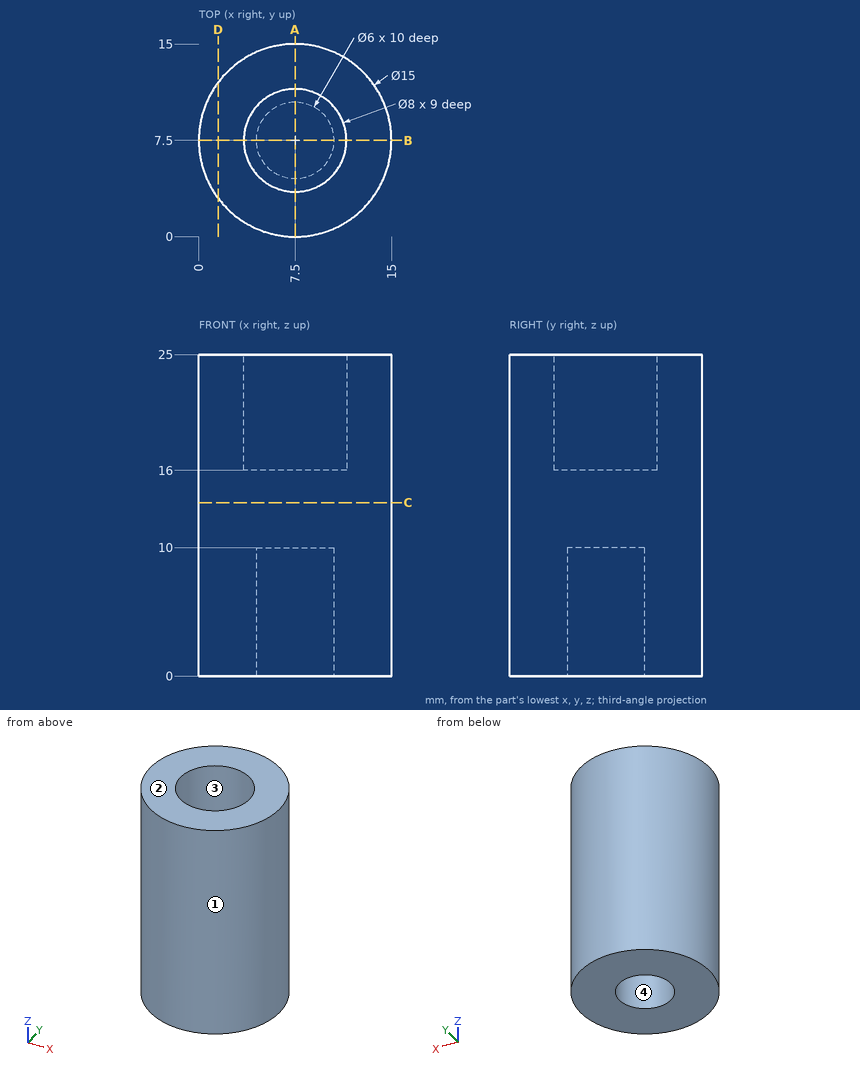
Design review of the part shown in the three views and the two pictorial views. Dimensions are in mm from the part's minimum x, y and z. Give positions to 0.01 mm unless a question says otherwise; leave off trailing zeros. Write each loop counter-clockwise with the first axis right and the second up, starting at its lowest first coordinate (ties: lowest second). Pieces come first, ordered by that corner, then holes. Notation, with made-up numbers: (47, 44) - (99, 44) arc R16 cw to (99, 56) - close; hole circle Ø6 at (39.25, 39). An arc over 180 degrees is marked (long way). Return JSON: item names as keys, results as strings. Group by question number.
(1) Insertion check: pin 1 (1 mm diameter, centred on x = 10, y = 13, fed in from -Z); pin 2 (2.5 mm diameter, centred on x = 7.5, y = 7.5, fed in from +Z); pin 3 (5.5 mm diameter, centred on x = 7.5, y = 7.5, fed in from -Z); pin 4 (5 mm diameter, centred on x = 3.5, z = 13.5, fed in from -Y). Each pin has a flat end and moves straight along its axis. Give the tip position at first contact, or say it passes through.
(2) We need section A-A, the plane x = 7.5. Give the boundary of the cut face in (y, z).
(3) We need section C-C, the plane z = 13.5. Give the boundary of the cut face in (x, y).
(4) We need section D-D, the plane x = 1.5. Give the boundary of the cut face in (y, z).
(5) Mouldability with a two-part tool opening along Y and no side actions: class the marked faces 1, 2, 3 and 4 as +Y half, -Y half, draft (parallel to the pull), parting line (faces both ways), or undercut.
(6) To check wall thickness, follow probe 1 along Y at (x, z) = (7.5, 2.75); probe 2 along Y at (x, z) = (9.75, 7.5); probe 3 along Z at (x, y) = (3.75, 7.75). State the ranges of each line that lie inside material, in increasing order.
Reported:
{
 "1": {"pin 1": "stops at z = 0", "pin 2": "stops at z = 16", "pin 3": "stops at z = 10", "pin 4": "stops at y = 0.15"},
 "2": {"outline": "(0, 0) - (4.5, 0) - (4.5, 10) - (10.5, 10) - (10.5, 0) - (15, 0) - (15, 25) - (11.5, 25) - (11.5, 16) - (3.5, 16) - (3.5, 25) - (0, 25) - close"},
 "3": {"outline": "circle Ø15 at (7.5, 7.5)"},
 "4": {"outline": "(3, 0) - (12, 0) - (12, 25) - (3, 25) - close"},
 "5": {"face 1": "parting line", "face 2": "draft", "face 3": "undercut", "face 4": "undercut"},
 "6": {"probe 1": "y = 0 to 4.5, 10.5 to 15", "probe 2": "y = 0.35 to 5.52, 9.48 to 14.65", "probe 3": "z = 0 to 16"}
}
